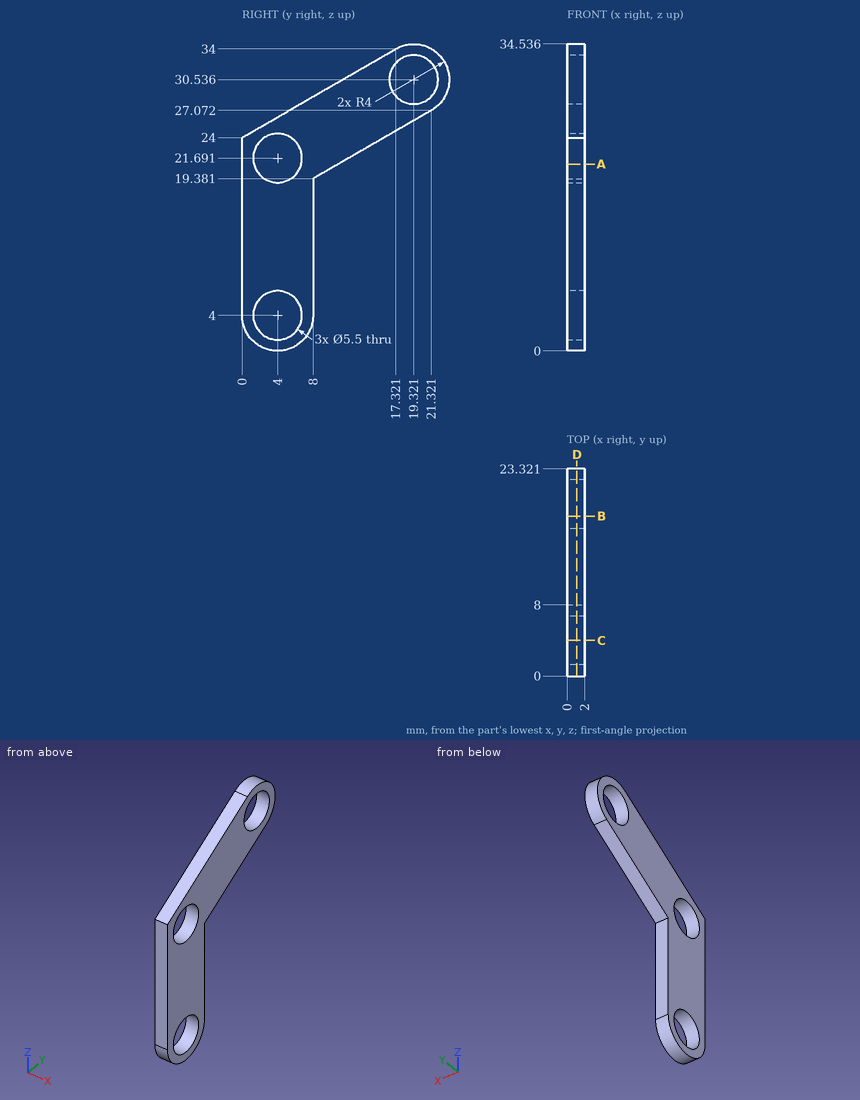
The drawing under review shows one solid part. Ordinate dimensions are in mm from its lowest x, y, z. Give positions to 0.01 mm unless a question says otherwise; leave off trailing zeros. Order: outer loops, then holes, each group sorted by start corner. A loop starts at its lowest first (then second) coordinate and runs counter-clockwise, first axis right, second up. Notation, with made-up numbers: (24.25, 70.5) - (71.25, 70.5) arc R25 cw to (71.25, 101.5) - close; hole circle Ø1 at (19, 6.25). An arc over 180 degrees is marked (long way). Answer as a JSON object with one key per item and string values. Group by question number.
Item 1: Take a section at D-D on x = 1.1. Give the number of separate pieces and of enclosed holes in the cut face, and give its area (3 significant figures).
Item 2: Take a section at B-B on y = 18. Give the boundary of the cut face in (x, z) (1 decimal).
Item 3: Clearance check with flat-ended pins moving along their axes: pin 1 Ø4.5 at (y, z) = (4, 4) entering from +X; pin 2 Ø1 at (x, y) = (1.5, 10) entering from -Z; pin 3 Ø0.6 at (x, z) = (1, 14) entering from +Y. State where each tip first meets the part, or that it passes through.
Item 4: Take a section at C-C on y = 4. Give the boundary of the cut face in (x, z).
Item 5: Wall thickness on line 1 along Y through (x, z) = (1.05, 4); line 2 along Z through (x, y) = (0.85, 6.25) (1 decimal); line 3 along Z through (x, y) = (0.25, 3) (1 decimal): over which ranges is each line inside the solid? List them lowest first.
Item 6: Take a section at A-A on z = 21. Give the boundary of the cut face in (x, y).
Reported:
{
 "1": {"separate pieces": "1", "enclosed holes": "3", "area": "262 mm^2"},
 "2": {"outline": "(0, 25.2) - (2, 25.2) - (2, 28.1) - (0, 28.1) - close; (0, 32.9) - (2, 32.9) - (2, 34.3) - (0, 34.3) - close"},
 "3": {"pin 1": "through", "pin 2": "z = 20.25", "pin 3": "y = 8"},
 "4": {"outline": "(0, 0) - (2, 0) - (2, 1.25) - (0, 1.25) - close; (0, 6.75) - (2, 6.75) - (2, 18.94) - (0, 18.94) - close; (0, 24.44) - (2, 24.44) - (2, 26.31) - (0, 26.31) - close"},
 "5": {"line 1": "0 to 1.25, 6.75 to 8", "line 2": "0.7 to 2.4, 5.6 to 20.1, 23.3 to 27.6", "line 3": "0.1 to 1.4, 6.6 to 19.1, 24.3 to 25.7"},
 "6": {"outline": "(0, 0) - (2, 0) - (2, 1.34) - (0, 1.34) - close; (0, 6.66) - (2, 6.66) - (2, 10.8) - (0, 10.8) - close"}
}
